Can you work these out from the drawing? Everything is in mm from the part's minimum corner. A direction names the side the tool comes from. Give positions to 0.01 mm unless a question says otherwise; leave off trailing zeros. Loops run counter-clockwise (first coordinate to the right, second up) from the corner with the lowest first, then second, coordinate; pieces in that order, holes last. Notation, with made-up numbers: (-39, 32.5) -> (-8, 32.5) arc R20 cw to (-8, 66.5) -> close; hole circle Ø10 at (68, -3). An arc over 180 degrees is marked (long way). Write item = value, one per line. Start each with the question number.
1) I want a section at D-D (z = 52). List the corners of the cut face in (x, y) for me, and give its area (3 significant figures).
2) On a 3-axis mill with a long thin cutter (end or side, diameter ignored), from which of +Z, -Z, +X, -X, +Y, -Y can I reach the whole of each face in a straight line? I mean the marked faces 1 and 2. Say none if no direction works.
3) I'm going to push flat-ended pins straight in: pin 1 Ø6 at (x, y) = (48.5, 53) entering from -Z; pin 2 Ø8 at (x, z) = (52, 5) entering from +Y; pin 3 Ø12 at (x, z) = (48, 54.5) entering from -Y. Where does each tip first touch, or does it pass through?
4) I want a section at B-B (z = 28.5). List the corners of the cut face in (x, y) for me.
5) I need wall thicknesses on probe 1 along X at (y, z) = (3, 52); probe 2 along Y at (x, z) = (48.5, 58.15); probe 3 along X at (y, z) = (0.9, 28.5). Which ranges of each line are inside material? Lowest first, please. Write a range as from..to.
6) I want a section at C-C (x = 53.5). List the corners of the cut face in (y, z) for me.
7) I want a section at A-A (x = 21). List the corners of the cut face in (y, z) for me, and give its area (3 significant figures).
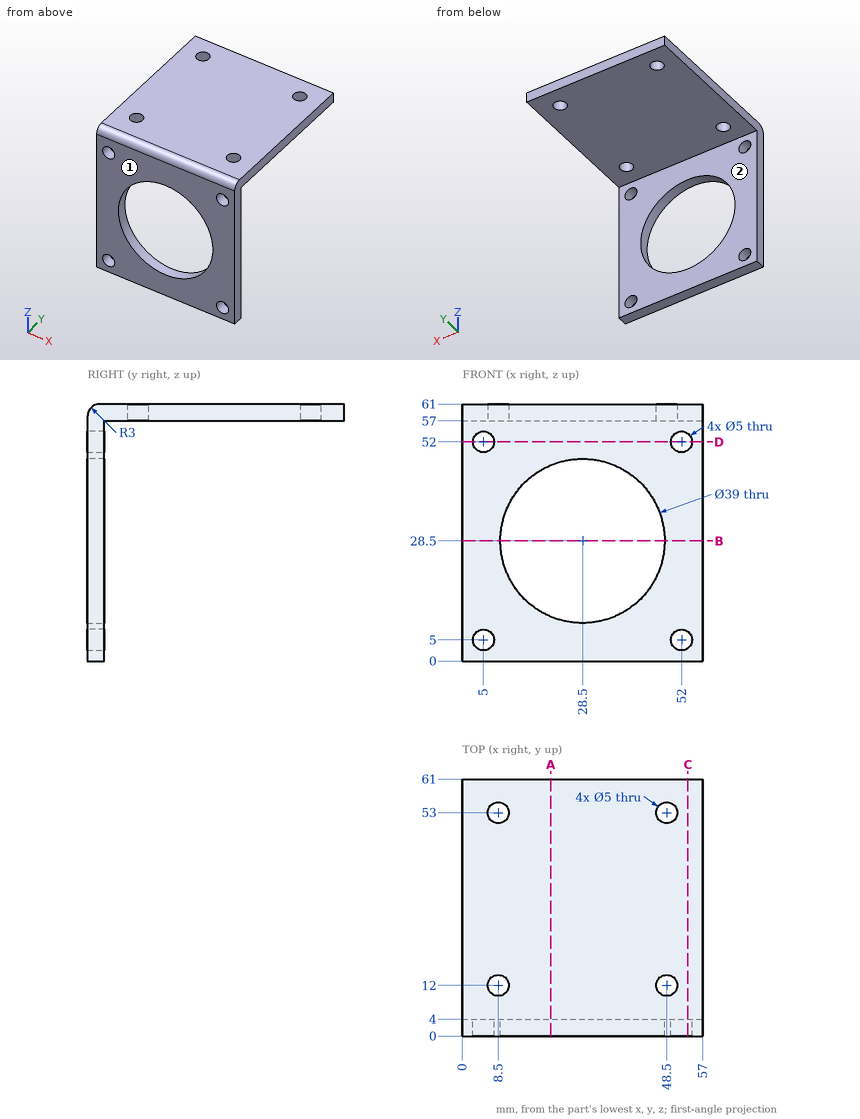
Answer list:
q1.outline = (0, 0) -> (2.5, 0) -> (2.5, 4) -> (0, 4) -> close; (7.5, 0) -> (49.5, 0) -> (49.5, 4) -> (7.5, 4) -> close; (54.5, 0) -> (57, 0) -> (57, 4) -> (54.5, 4) -> close
q1.area = 188 mm^2
q2.face_1 = +Z, -Z, +X, -X, -Y
q2.face_2 = -Z, +X, -X, +Y
q3.pin_1 = 57
q3.pin_2 = 4
q3.pin_3 = 0
q4.outline = (0, 0) -> (9, 0) -> (9, 4) -> (0, 4) -> close; (48, 0) -> (57, 0) -> (57, 4) -> (48, 4) -> close
q5.probe_1 = 0..2.5, 7.5..49.5, 54.5..57
q5.probe_2 = 0..9.5, 14.5..50.5, 55.5..61
q5.probe_3 = 0..9, 48..57
q6.outline = (0, 0) -> (4, 0) -> (4, 3) -> (0, 3) -> close; (0, 7) -> (4, 7) -> (4, 50) -> (0, 50) -> close; (0, 54) -> (4, 54) -> (4, 57) -> (61, 57) -> (61, 61) -> (3, 61) arc R3 ccw to (0, 58) -> close
q7.outline = (0, 0) -> (4, 0) -> (4, 10.5) -> (0, 10.5) -> close; (0, 46.5) -> (4, 46.5) -> (4, 57) -> (61, 57) -> (61, 61) -> (3, 61) arc R3 ccw to (0, 58) -> close
q7.area = 326 mm^2
